Geometry: final body of the model. Coordinates: model frame, mm. A direction names the side the tool comes from. Give positions to 0.01 mm unless a question says otherwise; leave off trailing zeros. Write each loop counter-clockwise with the first axis right and the second up, starting at its lowest first coordinate (ties: lowest second). Pieces come first, ordered by that corner, then holes. Notation, with made-up numbers: M 70.25,63.5 L 98.25,63.5 A16 ccw 98.25,89.5 Z; hole C 24.5,-28 d6. An arc over 180 degrees is marked long. Use a Markdown table: item, result. Add a question column.
(1) Pin query (flat end, axial travel): pin 1 Ø13 at (x, y) = (-0.5, 11.5) entering from +Z; pin 2 Ø5 at (y, z) = (-3, -3.5) entering from +X; pin 3 Ø3.5 at (x, y) = (3, 12.5) entering from -Z; pin 4 Ø8 at (y, z) = (9.5, 1.5) entering from -X. Return the tip coordinate at first contact, or that it passes through.
(2) Material intervals for L1, parallel to Y at x = 0, z = -5.5; L2, parallel to Z at x = 2.75, y = 4.75; L3, parallel to X at y = 8, z = -0.25, sorted ascending.
(3) Cut plane D-D (z = 6.5). Output: boundary loops of the cut face in (x, y).
(4) Cut plane C-C (z = 0). Output: boundary loops of the cut face in (x, y), plus the area to 3 significant figures.
(5) Reachability of faces 1 (the flat face through (-10, -5, 2)), 2 (the flat face through (0, 14, 9.22)), 3 (the flat face through (6, 9, -5)), 4 (the cylindrical face through (10, -5, 0)), 5 (the cylindrical face through (4.483, 10.412, 6.153)) from +Z, -Z, +X, -X, +Y, -Y: full face, straight path, thin tool, end or side. Return the list, or none.
(6) Draft query along Z for faces 6 (the flat face through (0, 14, -9.22)), 7 (the flat face through (-10, -5, -2)), 8 (the flat face through (0, 2, 0)), 9 (the flat face through (0, 16, 4)). Return one class per face: released by +Z, released by -Z, zero draft, split by the parting line, or undercut.
(7) Cut plane B-B (y = 11). Output: boundary loops of the cut face in (x, z).
(8) Cut plane A-A (x = 0). Output: boundary loops of the cut face in (y, z), plus the area to 3 significant figures.
```python
from build123d import *

# Parameters (mm, degrees)
SKETCH2_W           = 3
SKETCH2_H           = 4
CUT_EXTRUDE2_DEPTH  = 10
SKETCH6_W           = 12
SKETCH6_H           = 14
CUT_EXTRUDE3_DEPTH  = 14
BOSS_EXTRUDE1_REACH = 32.299
SKETCH7_W           = 12
SKETCH7_H           = 6.219544457
CUT_EXTRUDE4_REACH  = 30.033
SKETCH8_R           = 4.7


with BuildPart() as part:
    # Sketch1 → Revolve1 (revolve)
    with BuildSketch(Plane.XY, mode=Mode.PRIVATE) as revolve1_sk:
        Polygon((0, 0), (0, 2), (-10, 2), (-10, 16), (-11, 16), (-11, -10), (-10, -10), (-10, 0), align=None)
    revolve(revolve1_sk.sketch.rotate(Axis((0, 0, 0), (0, 1, 0)), 270), axis=Axis((0, 0, 0), (0, 1, 0)))

    # Sketch2 → Cut-Extrude2 (cut)
    with BuildSketch(Plane.XZ.offset(10)):
        with Locations((-10, 0)):
            Rectangle(SKETCH2_W, SKETCH2_H)
    extrude(amount=-CUT_EXTRUDE2_DEPTH, mode=Mode.SUBTRACT)

    # Sketch6 → Cut-Extrude3 (cut)
    with BuildSketch(Plane(origin=(0, 16, 0), x_dir=(1, 0, 0), z_dir=(0, 1, 0))):
        with Locations((0, -10)):
            Rectangle(SKETCH6_W, SKETCH6_H)
        with Locations((0, 10)):
            Rectangle(SKETCH6_W, SKETCH6_H)
    extrude(amount=-CUT_EXTRUDE3_DEPTH, mode=Mode.SUBTRACT)

    # Sketch7 → Boss-Extrude1 (add, up to next)
    with BuildSketch(Plane(origin=(0, 16, 0), x_dir=(1, 0, 0), z_dir=(0, 1, 0)), mode=Mode.PRIVATE) as boss_extrude1_sk1:
        with Locations((0, 6.109772229)):
            Rectangle(SKETCH7_W, SKETCH7_H)
    boss_extrude1_tool1 = extrude(boss_extrude1_sk1.sketch, amount=-BOSS_EXTRUDE1_REACH, mode=Mode.PRIVATE) - part.part
    # Sketch7 → Boss-Extrude1 (add, up to next)
    with BuildSketch(Plane(origin=(0, 16, 0), x_dir=(1, 0, 0), z_dir=(0, 1, 0)), mode=Mode.PRIVATE) as boss_extrude1_sk2:
        with Locations((0, -6.109772229)):
            Rectangle(SKETCH7_W, SKETCH7_H)
    boss_extrude1_tool2 = extrude(boss_extrude1_sk2.sketch, amount=-BOSS_EXTRUDE1_REACH, mode=Mode.PRIVATE) - part.part
    add(boss_extrude1_tool1.solids().sort_by_distance((0, 16, -6.109772))[0])
    add(boss_extrude1_tool2.solids().sort_by_distance((0, 16, 6.109772))[0])

    # Cut-Extrude4: up to this face of the body (flat: up to its plane)
    cut_extrude4_end = Plane(part.part.faces().sort_by_distance((0, 9, -9.219544457))[0])
    # Sketch8 → Cut-Extrude4 (cut, up to the picked face)
    with BuildSketch(Plane.XY.offset(9.219544457), mode=Mode.PRIVATE) as cut_extrude4_sk1:
        with Locations((0, 9)):
            Circle(SKETCH8_R)
    cut_extrude4_tool1 = split(extrude(cut_extrude4_sk1.sketch, amount=-CUT_EXTRUDE4_REACH, mode=Mode.PRIVATE), bisect_by=cut_extrude4_end, keep=Keep.BOTH, mode=Mode.PRIVATE)
    add(cut_extrude4_tool1.solids().sort_by(Axis((0, 9, 9.219544), (0, 0, -1)))[0], mode=Mode.SUBTRACT)


solid = part.part
```
Answer list:
| question | item | result |
|---|---|---|
| 1 | pin 1 | z = 9.22 |
| 1 | pin 2 | x = 10.95 |
| 1 | pin 3 | z = -9.22 |
| 1 | pin 4 | x = -11 |
| 2 | L1 | 0 to 4.3, 13.7 to 16 |
| 2 | L2 | -9.22 to -3, 3 to 9.22 |
| 2 | L3 | -11 to -10, 10 to 11 |
| 3 | outline | M -8.87,-10 L -7.6,-10 L -7.6,0 L 7.6,0 L 7.6,-10 L 8.87,-10 L 8.87,16 L 7.6,16 L 7.6,2 L 6,2 L 6,16 L -6,16 L -6,2 L -7.6,2 L -7.6,16 L -8.87,16 Z; hole C 0,9 d9.4 |
| 4 | outline | M -11,0 L 10,0 L 10,-10 L 11,-10 L 11,16 L 10,16 L 10,2 L -10,2 L -10,16 L -11,16 Z |
| 4 | area | 82.0 mm² |
| 5 | face 1 | -X, -Y |
| 5 | face 2 | +Z, +X, -X, +Y |
| 5 | face 3 | +Y |
| 5 | face 4 | -Y |
| 5 | face 5 | +Z, -Z |
| 6 | face 6 | released by -Z |
| 6 | face 7 | undercut |
| 6 | face 8 | undercut |
| 6 | face 9 | zero draft |
| 7 | outline | M -6,-9.22 L -4.25,-9.22 L -4.25,-3 L -6,-3 L -6,-8 A10 cw -6,8 L -6,3 L -4.25,3 L -4.25,9.22 L -6,9.22 A11 ccw Z; M 4.25,-9.22 L 6,-9.22 A11 ccw 6,9.22 L 4.25,9.22 L 4.25,3 L 6,3 L 6,8 A10 cw 6,-8 L 6,-3 L 4.25,-3 Z |
| 8 | outline | M -10,-11 L 2,-11 L 2,-9.22 L 4.3,-9.22 L 4.3,-3 L 2,-3 L 2,3 L 4.3,3 L 4.3,9.22 L 2,9.22 L 2,11 L -10,11 L -10,10 L 0,10 L 0,-10 L -10,-10 Z; M 13.7,-9.22 L 16,-9.22 L 16,-3 L 13.7,-3 Z; M 13.7,3 L 16,3 L 16,9.22 L 13.7,9.22 Z |
| 8 | area | 121 mm² |
